```python
from build123d import *

# Parameters (mm, degrees)
SKETCH1_W               = 8
SKETCH1_H               = 8
BOSS_EXTRUDE1_DEPTH     = 3
CUT_EXTRUDE1_DEPTH      = 12.704699911
CUT_EXTRUDE1_DEPTH_BACK = 12.704699911
CUT_EXTRUDE2_DEPTH      = 11
SKETCH4_R               = 1.75
CUT_EXTRUDE3_DEPTH      = 0.4
SKETCH5_W               = 8
SKETCH5_H               = 1
BOSS_EXTRUDE2_DEPTH     = 2
FILLET1_R               = 4
CUT_EXTRUDE4_DEPTH      = 0.4


with BuildPart() as part:
    # Sketch1 → Boss-Extrude1 (new body)
    with BuildSketch(Plane(origin=(0, 0, 0), x_dir=(1, 0, 0), z_dir=(0, 1, 0))):
        with Locations((4, 4)):
            Rectangle(SKETCH1_W, SKETCH1_H)
    extrude(amount=BOSS_EXTRUDE1_DEPTH)

    # Sketch2 → Cut-Extrude1 (cut, two sides: drawn at the far end of the back side and taken through both)
    with BuildSketch(Plane.XY.offset(-CUT_EXTRUDE1_DEPTH_BACK)):
        Polygon((0, 0), (0.6, 3), (0, 3), align=None)
        Polygon((8, 0), (7.4, 3), (8, 3), align=None)
    extrude(amount=CUT_EXTRUDE1_DEPTH + CUT_EXTRUDE1_DEPTH_BACK, mode=Mode.SUBTRACT)

    # Sketch3 → Cut-Extrude2 (cut)
    with BuildSketch(Plane(origin=(0, 0, 0), x_dir=(0, 0, -1), z_dir=(1, 0, 0))):
        Polygon((0, 0), (0.6, 3), (0, 3), align=None)
        Polygon((8, 3), (7.4, 3), (8, 0), align=None)
    extrude(amount=CUT_EXTRUDE2_DEPTH, mode=Mode.SUBTRACT)

    # Sketch4 → Cut-Extrude3 (cut)
    with BuildSketch(Plane.XZ):
        with Locations(Location((4, -3.75, 0), (0, 0, 270))):
            Circle(SKETCH4_R)
    extrude(amount=-CUT_EXTRUDE3_DEPTH, mode=Mode.SUBTRACT)

    # Sketch5 → Boss-Extrude2 (add)
    with BuildSketch(Plane.XZ):
        with Locations((4, -7.5)):
            Rectangle(SKETCH5_W, SKETCH5_H)
    extrude(amount=BOSS_EXTRUDE2_DEPTH)

    # Fillet1
    # the kernel refuses this fillet: 4 mm, written as the material it takes off along each edge
    with BuildSketch(Plane(origin=(8, -2, -16.660254038), x_dir=(0, 1, 0), z_dir=(0, 0, 1)), Plane(origin=(0, -2, 1.660254038), x_dir=(0, 1, 0), z_dir=(0, 0, -1))) as fillet1_piece_1:
        with BuildLine():
            CenterArc((4, 3.464101615), FILLET1_R, 180, 60)
            Line((0, 3.464101615), (-0.08, 3.464101615))
            Line((-0.08, 3.464101615), (-0.08, 0))
            Line((-0.08, 0), (0, -0.08))
            ThreePointArc((0, -0.08), (1, -0.08), (1.96, -0.069282032))
            Line((1.96, -0.069282032), (2, 0))
        make_face()
    extrude(amount=18.320508076, mode=Mode.SUBTRACT)

    # Sketch6 → Cut-Extrude4 (cut)
    with BuildSketch(Plane(origin=(0, 3, 0), x_dir=(1, 0, 0), z_dir=(0, 1, 0))):
        Polygon((3.039241423, 1.586469201), (4.258191744, 6.586469201), (4.982350398, 6.586469201), (3.76440168, 1.586469201), align=None)
    extrude(amount=-CUT_EXTRUDE4_DEPTH, mode=Mode.SUBTRACT)


solid = part.part
```
For this review, take the finished solid that the model builds, in its own axes (mm). A direction names the side the tool comes from. Give positions to 0.01 mm unless a question says otherwise; leave off trailing zeros. Loops run counter-clockwise (first coordinate to the right, second up) from the corner with the lowest first, then second, coordinate; pieces in that order, holes last. Notation, with made-up numbers: M -2.75,-32.75 L 44.25,-32.75 A19 ccw 44.25,-18.75 Z; hole C 49,76.5 d10. An arc over 180 degrees is marked long. One line per item, written item: value. Start each with the question number.
Q1. Add section C-C (y = 0.9). Give the boundary of the cut face in (x, z).
Q2. Add section A-A (x = 7.25). Give the boundary of the cut face in (y, z), and give its area (3 significant figures).
Q3. Machinability: for faces 4 (the face through (7.7, 1.5, -4.1)), 5 (the face through (4, 0.4, -4)), 6 (the face through (3, 0, -2)), 7 (the face through (4, 2.6, -4)), which of the approach directions +Z, -Z, +X, -X, +Y, -Y give a long, thin tool a straight path to every point of the face, cutting with its end or side? Answer none if there is none.
Q4. Add section B-B (z = -3.75). Give the boundary of the cut face in (x, y), and give its area (3 significant figures).
Q5. Clearance check with flat-ended pins moving along their axes: pin 1 Ø2 at (x, z) = (5, -2.5) entering from -Y; pin 2 Ø1.5 at (x, z) = (4.5, -4.5) entering from -Y; pin 3 Ø2 at (x, y) = (2.5, -0.5) entering from +Z; pin 4 Ø2 at (x, y) = (3, 2.5) entering from -Z. State where each tip first meets the part, or that it passes through.
Q6. For L1, parallel to Y at x = 2.25, z = -1.5; L2, parallel to X at y = 0.25, z = -3.75; L3, parallel to Z at x = 2.75, y = -1.5, list the stretches that pass through material, from the lowest coordinate up.
Q7. Add section D-D (x = 1.5). Give the boundary of the cut face in (y, z), and give its area (3 significant figures).
Q8. Draft analysis for pull direction Z (two halves, no side actions). For faces 1 (the face through (4, -1, -8)), 2 (the face through (3, 3, -4)), 3 (the face through (3.64, 2.8, -4.05)), state which applies: released by +Z, released by -Z, zero draft, split by the parting line, or undercut.
Reply:
1. outline: M 0.18,-7.82 L 7.82,-7.82 L 7.82,-0.18 L 0.18,-0.18 Z
2. outline: M -0.94,-8 L 0,-8 L 3,-7.4 L 3,-0.6 L 0,0 L 0,-7 L -0.94,-7 Z
2. area: 23.1 mm²
3. face 4: +Z, -Z, +X, +Y
3. face 5: -Y
3. face 6: +Z, +X, -X, -Y
3. face 7: +Y
4. outline: M 0,0 L 2.25,0 L 2.25,0.4 L 5.75,0.4 L 5.75,0 L 8,0 L 7.4,3 L 4.29,3 L 4.29,2.6 L 3.57,2.6 L 3.57,3 L 0.6,3 Z
4. area: 20.5 mm²
5. pin 1: y = 0
5. pin 2: y = 0.4
5. pin 3: z = 0
5. pin 4: z = -7.7
6. L1: 0 to 3
6. L2: 0.05 to 2.25, 5.75 to 7.95
6. L3: -8 to -7
7. outline: M -1.48,-8 L 0,-8 L 3,-7.4 L 3,-0.6 L 0,0 L 0,-7 L -1.48,-7 Z
7. area: 23.7 mm²
8. face 1: released by -Z
8. face 2: zero draft
8. face 3: undercut
